Read the model definition and answer for the solid it produces. Units are mm, in the model's axes. Face numbers are marked on the shaded views. A direction names the side the tool comes from. Coordinates: 2 decimals unless noted, no trailing zeros. Loops run counter-clockwise (first coordinate to the right, second up) from the corner with the lowest first, then second, coordinate; pieces in that order, holes last.
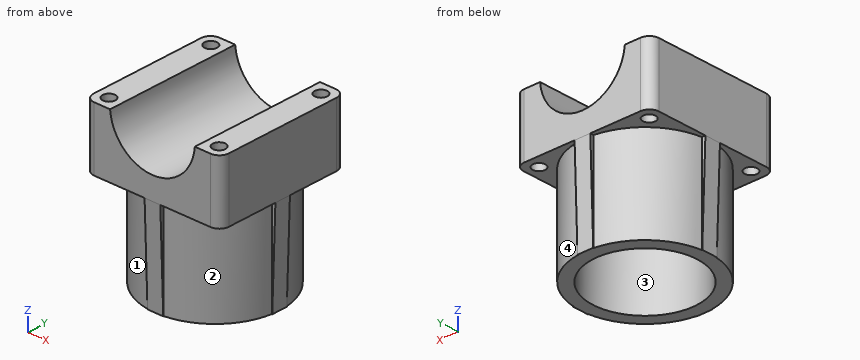
from build123d import *

# Parameters (mm, degrees)
CROQUIS1_W              = 43
CROQUIS1_H              = 43
SALIENTE_EXTRUIR1_DEPTH = 19.5
CROQUIS2_R              = 13.5
CORTAR_EXTRUIR1_DEPTH   = 44
CROQUIS3_R              = 2
CORTAR_EXTRUIR2_DEPTH   = 20.5
REDONDEO1_R             = 3
CROQUIS5_R              = 20.5
CROQUIS5_R_2            = 16.5
SALIENTE_EXTRUIR2_DEPTH = 30
EXTRUIR_L_MINA1_REACH   = 45.626
CROQUIS7_W              = 5
CROQUIS7_H              = 30.01666204
EXTRUIR_L_MINA2_REACH   = 45.626
CROQUIS8_W              = 30.01666204
CROQUIS8_H              = 5
EXTRUIR_L_MINA3_REACH   = 45.626
CROQUIS9_W              = 5
CROQUIS9_H              = 30.016662039
EXTRUIR_L_MINA4_REACH   = 45.626
CROQUIS10_W             = 30.016662039
CROQUIS10_H             = 5


with BuildPart() as part:
    # Croquis1 → Saliente-Extruir1 (new body)
    with BuildSketch(Plane.XY):
        with Locations((-58.504320503, 22.141791045)):
            Rectangle(CROQUIS1_W, CROQUIS1_H)
    extrude(amount=SALIENTE_EXTRUIR1_DEPTH)

    # Croquis2 → Cortar-Extruir1 (cut, through all)
    with BuildSketch(Plane(origin=(0, 43.641791045, 0), x_dir=(1, 0, 0), z_dir=(0, 1, 0))):
        with Locations((-58.504320503, -20.5)):
            Circle(CROQUIS2_R)
    extrude(amount=-CORTAR_EXTRUIR1_DEPTH, mode=Mode.SUBTRACT)

    # Croquis3 → Cortar-Extruir2 (cut, through all)
    with BuildSketch(Plane.XY.offset(19.5)):
        with Locations((-76.004320503, 39.641791045)):
            Circle(CROQUIS3_R)
        with Locations((-41.004320503, 39.641791045)):
            Circle(CROQUIS3_R)
        with Locations((-41.004320503, 4.641791045)):
            Circle(CROQUIS3_R)
        with Locations((-76.004320503, 4.641791045)):
            Circle(CROQUIS3_R)
    extrude(amount=-CORTAR_EXTRUIR2_DEPTH, mode=Mode.SUBTRACT)

    # Redondeo1
    redondeo1_edges = [part.edges().sort_by_distance(p)[0] for p in [
        (-80.004320503, 43.641791045, 9.75),
        (-37.004320503, 43.641791045, 9.75),
        (-37.004320503, 0.641791045, 9.75),
        (-80.004320503, 0.641791045, 9.75),
    ]]
    fillet(redondeo1_edges, radius=REDONDEO1_R)

    # Croquis5 → Saliente-Extruir2 (add)
    with BuildSketch(Plane(origin=(0, 0, 0), x_dir=(-1, 0, 0), z_dir=(0, 0, -1))):
        with Locations((58.504320503, 22.141791045)):
            Circle(CROQUIS5_R)
        with Locations((58.504320503, 22.141791045)):
            Circle(CROQUIS5_R_2, mode=Mode.SUBTRACT)
    extrude(amount=SALIENTE_EXTRUIR2_DEPTH)

    # Croquis7 → Extruir-Lámina1 (add, up to next)
    with BuildSketch(Plane(origin=(0, 43.593353985, -1.453111799), x_dir=(-1, 0, 0), z_dir=(0, -0.999444907, 0.03331483)), mode=Mode.PRIVATE) as extruir_l_mina1_sk1:
        with Locations((58.504320503, 13.55441216)):
            Rectangle(CROQUIS7_W, CROQUIS7_H)
    extruir_l_mina1_tool1 = extrude(extruir_l_mina1_sk1.sketch, amount=EXTRUIR_L_MINA1_REACH, mode=Mode.PRIVATE) - part.part
    add(extruir_l_mina1_tool1.solids().sort_by_distance((-58.504321, 43.141791, -15))[0])

    # Croquis8 → Extruir-Lámina2 (add, up to next)
    with BuildSketch(Plane(origin=(-36.963250225, 0, 1.232108341), x_dir=(0.03331483, 0, 0.999444907), z_dir=(-0.999444907, 0, 0.03331483)), mode=Mode.PRIVATE) as extruir_l_mina2_sk1:
        with Locations((-16.241123675, 22.141791045)):
            Rectangle(CROQUIS8_W, CROQUIS8_H)
    extruir_l_mina2_tool1 = extrude(extruir_l_mina2_sk1.sketch, amount=EXTRUIR_L_MINA2_REACH, mode=Mode.PRIVATE) - part.part
    add(extruir_l_mina2_tool1.solids().sort_by_distance((-37.504321, 22.141791, -15))[0])

    # Croquis9 → Extruir-Lámina3 (add, up to next)
    with BuildSketch(Plane(origin=(0, 0.641078735, 0.021369291), x_dir=(1, 0, 0), z_dir=(0, 0.999444907, 0.03331483)), mode=Mode.PRIVATE) as extruir_l_mina3_sk1:
        with Locations((-58.504320503, 15.02971218)):
            Rectangle(CROQUIS9_W, CROQUIS9_H)
    extruir_l_mina3_tool1 = extrude(extruir_l_mina3_sk1.sketch, amount=EXTRUIR_L_MINA3_REACH, mode=Mode.PRIVATE) - part.part
    add(extruir_l_mina3_tool1.solids().sort_by_distance((-58.504321, 1.141791, -15))[0])

    # Croquis10 → Extruir-Lámina4 (add, up to next)
    with BuildSketch(Plane(origin=(-79.915525474, 0, -2.663850849), x_dir=(0.03331483, 0, -0.999444907), z_dir=(0.999444907, 0, 0.03331483)), mode=Mode.PRIVATE) as extruir_l_mina4_sk1:
        with Locations((12.343000664, 22.141791045)):
            Rectangle(CROQUIS10_W, CROQUIS10_H)
    extruir_l_mina4_tool1 = extrude(extruir_l_mina4_sk1.sketch, amount=EXTRUIR_L_MINA4_REACH, mode=Mode.PRIVATE) - part.part
    add(extruir_l_mina4_tool1.solids().sort_by_distance((-79.504321, 22.141791, -15))[0])


solid = part.part
Q1. A cutting plane is placed at D-D (y = 35). Give the vertices of the cut face in (x, z), then the cut area to 3 significant figures.
Findings below:
outline: (-80, 0) - (-74.47, 0) - (-74.47, -30) - (-68.84, -30) - (-68.84, 0) - (-48.16, 0) - (-48.16, -30) - (-42.54, -30) - (-42.54, 0) - (-37, 0) - (-37, 19.5) - (-45.04, 19.5) arc R13.5 cw to (-71.97, 19.5) - (-80, 19.5) - close
area: 917 mm2
Q2. A cutting plane is placed at A-A (z = 12.5). Give the vertices of the cut face in (x, y).
Findings below:
outline: (-80, 3.64) arc R3 ccw to (-77, 0.64) - (-69.38, 0.64) - (-69.38, 43.64) - (-77, 43.64) arc R3 ccw to (-80, 40.64) - close; (-47.63, 0.64) - (-40, 0.64) arc R3 ccw to (-37, 3.64) - (-37, 40.64) arc R3 ccw to (-40, 43.64) - (-47.63, 43.64) - close; hole circle Ø4 at (-76, 4.64); hole circle Ø4 at (-76, 39.64); hole circle Ø4 at (-41, 4.64); hole circle Ø4 at (-41, 39.64)
Q3. Flat-ended cylindrical pins translate along their axes: pin 1 Ø5 at (x, y) = (-41, 39.64) entering from -Z; pin 2 Ø8 at (x, y) = (-64.5, 29.5) entering from +Z; pin 3 Ø1.5 at (x, z) = (-65, -21.5) entering from -Y. Find the tip coordinate at first contact, or state that the pin passes through.
Findings below:
pin 1: stops at z = 0
pin 2: stops at z = 11.43
pin 3: stops at y = 2.46
Q4. A cutting plane is placed at C-C (x = -67.5). Give the vertices of the cut face in (y, z), then the cut area to 3 significant figures.
Findings below:
outline: (0.64, 0) - (3.72, 0) - (3.72, -30) - (8.31, -30) - (8.31, 0) - (35.97, 0) - (35.97, -30) - (40.56, -30) - (40.56, 0) - (43.64, 0) - (43.64, 10.43) - (0.64, 10.43) - close
area: 724 mm2
Q5. Which of the six approach directions +Z, -Z, +X, -X, +Y, -Y give full straight-line access (tool end or side, diameter ignored) to the marked faces 1, 2, 3 and 4?
Findings below:
face 1: -Z, -X, -Y
face 2: -Z, +X, -Y
face 3: -Z
face 4: -Z, +X, +Y
Q6. A cutting plane is placed at B-B (z = 3.5). Give the vertices of the cut face in (x, y).
Findings below:
outline: (-80, 3.64) arc R3 ccw to (-77, 0.64) - (-40, 0.64) arc R3 ccw to (-37, 3.64) - (-37, 40.64) arc R3 ccw to (-40, 43.64) - (-77, 43.64) arc R3 ccw to (-80, 40.64) - close; hole circle Ø4 at (-76, 4.64); hole circle Ø4 at (-76, 39.64); hole circle Ø4 at (-41, 4.64); hole circle Ø4 at (-41, 39.64)
Q7. Straight lines are drawn through the part: probe 1 along Z at (x, y) = (-43.5, 25); probe 2 along X at (y, z) = (23, -18.5); probe 3 along Y at (x, z) = (-54.5, -26). For each, find the intervals that lie inside material, in ascending order.
Findings below:
probe 1: z = 0 to 19.5
probe 2: x = -79.39 to -74.98, -42.03 to -37.62
probe 3: y = 2.04 to 6.14, 38.15 to 42.25
